Solid Edge part; units mm, degrees
sketch "Sketch1" plane through (0, 0, 0) normal (0, -1, 0) x (1, 0, 0)
  circle A0 centre (-17.5, 0) radius 1.6
  line L0 (-20.75, -18.3456) -> (-20.75, 0)
  line L1 (-9, -18.3456) -> (-20.75, -18.3456)
  line L2 (-9, -11.0482) -> (-9, -18.3456)
  arc A1 (-14.25, 0) -> (-9, -11.0482) centre (0, 0) ccw
  arc A2 (-20.75, 0) -> (-14.25, 0) centre (-17.5, 0) cw
  arc A3 (9, -11.0482) -> (14.25, 0) centre (0, 0) ccw
  arc A4 (14.25, 0) -> (20.75, 0) centre (17.5, 0) cw
  line L3 (20.75, 0) -> (20.75, -18.3456)
  line L4 (20.75, -18.3456) -> (9, -18.3456)
  line L5 (9, -18.3456) -> (9, -11.0482)
  circle A5 centre (17.5, 0) radius 1.6
  dimension "D1" = 17.5
extrude "Protrusion1" add sketch "Sketch1" against normal blind 6.5
sketch "Sketch2" plane through (14.875, 3.25, -18.3456) normal (0, 0, -1) x (0, -1, 0)
  line L0 (3.25, 35.625) -> (-25.75, 35.625)
  line L1 (-25.75, 35.625) -> (-25.75, -44.375)
  line L2 (-25.75, -44.375) -> (-5.75, -44.375)
  line L3 (-5.75, -44.375) -> (-5.75, -5.875)
  line L4 (-5.75, -5.875) -> (3.25, -5.875)
  line L5 (3.25, -5.875) -> (3.25, 35.625)
  dimension "D1" = 3.25
  dimension "D2" = 25.75
  dimension "D3" = 25.75
  dimension "D4" = 3.25
extrude "ExtrudedProtrusion_3" add sketch "Sketch2" along normal blind 10
sketch "Sketch3" plane through (9.25, 14.5, -28.3456) normal (0, 0, -1) x (0, 1, 0)
  line L0 (-14.5, -6.25) -> (-10.5, -6.25)
  line L1 (-10.5, -6.25) -> (-10.5, -12.25)
  line L2 (-10.5, -12.25) -> (-14.5, -12.25)
  line L3 (-14.5, -12.25) -> (-14.5, -6.25)
  dimension "D1" = 14.5
  dimension "D2" = 10.5
extrude "ExtrudedCutout_1" cut sketch "Sketch3" against normal blind 45
sketch "Sketch4" plane through (-20.75, 14.5, -14.1728) normal (-1, 0, 0) x (0, 1, 0)
  line L0 (-8, 4.1728) -> (-8, -10.8272)
  line L1 (7, 4.1728) -> (-8, -10.8272)
  line L2 (-8, 4.1728) -> (7, 4.1728)
  dimension "D1" = 8
  dimension "D2" = 8
extrude "Protrusion2" add sketch "Sketch4" against normal up to vertex (41.5 mm away)
sketch "Sketch5" plane through (9.25, 19, -18.3456) normal (0, 0, 1) x (1, 0, 0)
  line L0 (-23.6435, -12.5) -> (-23.6435, 24.588)
  line L1 (-23.6435, 24.588) -> (5, 24.588)
  line L2 (5, 24.588) -> (5, -12.5)
  line L3 (5, -12.5) -> (-23.6435, -12.5)
extrude "ExtrudedCutout_2" cut sketch "Sketch5" along normal blind 110
sketch "Sketch6" plane through (19.25, 14.5, -18.3456) normal (0, 0, 1) x (-1, 0, 0)
  circle A0 centre (-35, -4.5) radius 1.6
  circle A1 centre (-15, -4.5) radius 1.6
extrude "Cutout1" cut sketch "Sketch6" against normal up to vertex (24.5 mm away)
chamfer "Letörés_1" distance 5 angle 45 11 edges at (19.25, 29, -28.3456) (-20.75, 29, -23.3456) (19.25, 29, -18.3456) (59.25, 29, -23.3456) (59.25, 9, -23.3456) (40, 9, -28.3456) (11.875, 0, -28.3456) (-11.875, 0, -28.3456) (40, 9, -18.3456) (-20.75, 14.5, -28.3456) (20.75, 4.5, -28.3456)
chamfer "Letörés_2" distance 1 angle 45 4 edges at (20.75, 14, -10.8456) (14.25, 14, -10.8456) (-14.3935, 14, -10.8456) (-20.75, 14, -10.8456)
chamfer "Letörés_3" distance 0.5 angle 45 4 edges at (35.85, 19, -28.3456) (35.85, 19, -18.3456) (55.85, 19, -28.3456) (55.85, 19, -18.3456)
chamfer "Letörés_4" distance 2 angle 45 4 edges at (3, 0, -20.8456) (3, 2, -25.3456) (-3, 2, -25.3456) (-3, 0, -20.8456)
CAD build for the part. Positions are in the model's coordinates, mm. A direction names the side the tool comes from. Round coordinates to 2 decimals unless told otherwise and drop trailing zeros. Loops run counter-clockwise (first coordinate to the right, second up) from the corner with the lowest first, then second, coordinate; pieces in that order, holes last. Notation, with made-up numbers: M -35,32 L -20,32 A24 ccw -20,69 Z; hole C 71.5,21 d6. An arc over 180 degrees is marked long. One line per question, with ' | ' between items. Start each with the question number.
Item 1: Wall check: line 1 (X direction, y = 19, z = -21); line 2 (X direction, y = 18, z = -18); line 3 (X direction, y = 19, z = -24.75). Give the ranges that are in metal, low to high.
Item 2: Cut at D-D, the plane z = -13.5. Write the cut outline in (x, y), plus the area to 3 significant figures.
Item 3: Cut at B-B, the plane y = 19. State how many separate pieces and enclosed holes the cut face has, plus the area to 3 significant figures.
Item 4: Cut at C-C, the plane z = -20. Write the cut outline in (x, y).
Item 5: Cut at A-A, the plane x = 34.25. Write the cut outline in (y, z), plus the area to 4 significant figures.
Item 6: Pin check, flat tips, straight feed: pin 1 Ø7 at (x, y) = (25.5, 12) entering from +Z; pin 2 Ø3 at (y, z) = (2.5, -13) entering from +X; pin 3 Ø6 at (x, z) = (15, -9) entering from +Y. Stop position of each tip, or through.
Item 7: Two-plate mould, pull along X, no slides. Class faces 4 (the flat face through (57.27, 25.98, -23.28)), 5 (the flat face through (40.27, 11.535, -20.811)), 6 (the cylindrical face through (-19.1, 3.2, 0.07)): pulls with the +X half, pulls with the -X half, needs draft (parallel to the pull), parting line crosses it, or undercut.
Item 8: Which spindle directions (+Z, -Z, +X, -X, +Y, -Y) get a long thin tool onto all of the face, cutting with end or side? Do faces 1 (the flat face through (4, 1, -21)), 2 (the cylindrical face through (-12.908, 3.204, -6.036)), 3 (the flat face through (-14, 6.5, -9)). Say none if no direction does.
Responses:
1) line 1: x = -20.75 to 32.65, 35.85 to 52.65, 55.85 to 59.25 | line 2: x = -20.75 to -14.39, 14.25 to 20.75 | line 3: x = -19.35 to 32.65, 35.85 to 52.65, 55.85 to 59.25
2) outline: M -20.75,0 L -9,0 L -9,6.5 L -14.39,6.5 L -14.39,15.24 L -15.39,16.65 L -19.75,16.65 L -20.75,15.24 Z; M 9,0 L 20.75,0 L 20.75,15.24 L 19.75,16.65 L 15.25,16.65 L 14.25,15.24 L 14.25,6.5 L 9,6.5 Z | area: 280 mm²
3) separate pieces: 3 | enclosed holes: 0 | area: 752 mm²
4) outline: M -20.75,0 L -5,0 L -3,2 L -3,4 L 3,4 L 3,2 L 5,0 L 20.75,0 L 20.75,12.35 L 57.6,12.35 L 59.25,14 L 59.25,24 L 57.6,25.65 L -19.1,25.65 L -20.75,24 Z; hole C 34.25,19 d3.2; hole C 54.25,19 d3.2
5) outline: M 9,-23.35 L 14,-28.35 L 16.9,-28.35 L 17.4,-27.85 L 17.4,-18.85 L 16.9,-18.35 L 14,-18.35 Z; M 20.6,-27.85 L 21.1,-28.35 L 24,-28.35 L 29,-23.35 L 24,-18.35 L 21.1,-18.35 L 20.6,-18.85 Z | area: 117.5 mm²
6) pin 1: stops at z = -18.35 | pin 2: stops at x = 20.75 | pin 3: stops at y = 15.14
7) face 4: pulls with the +X half | face 5: needs draft | face 6: undercut
8) face 1: +Z, -Z, -Y | face 2: +Z, +Y, -Y | face 3: +Z, +Y
